Could you check a few things on this model? Use its own coordinates, in mm. Round coordinates to 2 decimals unless told otherwise and drop trailing zeros. Loops run counter-clockwise (first coordinate to the right, second up) from the corner with the lowest first, then second, coordinate; pieces in that order, holes last. Notation, with made-up numbers: (89, 9) -> (94, 9) arc R29 ccw to (94, 30) -> close; hole circle Ø10 at (28, 34). An arc over 180 degrees is marked (long way). Write each question's results on one line, items separated by ' | '.
from build123d import *

# Parameters (mm, degrees)
SKETCH_W      = 12
SKETCH_H      = 45
PAD_DEPTH     = 5
SKETCH001_R   = 2.2
SKETCH001_R_2 = 2
POCKET_DEPTH  = 5.001
CHAMFER_SIZE2 = 12
CHAMFER_SIZE  = 3
FILLET_R      = 3
FILLET001_R   = 5.5


with BuildPart() as part:
    # Sketch → Pad (new body)
    with BuildSketch(Plane.XY):
        Rectangle(SKETCH_W, SKETCH_H)
    extrude(amount=PAD_DEPTH)

    # Sketch001 (on Face6 of Pad) → Pocket (cut, through all)
    with BuildSketch(Plane.XY.offset(5)):
        with Locations((0, 17)):
            Circle(SKETCH001_R)
        with Locations((-0.5, -16.5)):
            Circle(SKETCH001_R_2)
        with Locations((-0.5, -4.5)):
            Circle(SKETCH001_R_2)
    extrude(amount=-POCKET_DEPTH, mode=Mode.SUBTRACT)

    # Chamfer
    chamfer_edges = [part.edges().sort_by_distance(p)[0] for p in [
        (6, -22.5, 2.5),
    ]]
    chamfer_side = part.faces().sort_by_distance((0, -22.5, 2.5))[0]
    chamfer(chamfer_edges, length=CHAMFER_SIZE, length2=CHAMFER_SIZE2, reference=chamfer_side)

    # Fillet
    fillet_edges = [part.edges().sort_by_distance(p)[0] for p in [
        (3, -22.5, 2.5),
    ]]
    fillet(fillet_edges, radius=FILLET_R)

    # Fillet001
    fillet001_edges = [part.edges().sort_by_distance(p)[0] for p in [
        (6, 22.5, 2.5),
        (-6, 22.5, 2.5),
    ]]
    fillet(fillet001_edges, radius=FILLET001_R)


solid = part.part
1) I want a section at B-B, the plane z = 4.45. Write out the boundary of the cut face in (x, y), plus the area to 3 significant figures.
Model answer:
outline: (-6, -22.5) -> (0.66, -22.5) arc R3 ccw to (3.57, -20.23) -> (6, -10.5) -> (6, 17) arc R5.5 ccw to (0.5, 22.5) -> (-0.5, 22.5) arc R5.5 ccw to (-6, 17) -> close; hole circle Ø4 at (-0.5, -16.5); hole circle Ø4 at (-0.5, -4.5); hole circle Ø4.4 at (0, 17) | area: 468 mm2
2) I want a section at D-D, the plane x = 4.25. Write out the boundary of the cut face in (y, z).
Model answer:
outline: (-17.5, 0) -> (21.02, 0) -> (21.02, 5) -> (-17.5, 5) -> close
3) I need wall thicknesses on line 1 (Y direction, x = 0, z = 1.45); line 2 (Y direction, x = -0.5, z = 3.85); line 3 (X direction, y = -16, z = 4.4) (1 decimal). Which ranges of each line are inside material? Lowest first, please.
Model answer:
line 1: y = -22.5 to -18.44, -14.56 to -6.44, -2.56 to 14.8, 19.2 to 22.5 | line 2: y = -22.5 to -18.5, -14.5 to -6.5, -2.5 to 14.86, 19.14 to 22.5 | line 3: x = -6 to -2.4, 1.4 to 4.6
4) I want a section at A-A, the plane y = -16.5. Write out the boundary of the cut face in (x, z), plus the area to 3 significant figures.
Model answer:
outline: (-6, 0) -> (-2.5, 0) -> (-2.5, 5) -> (-6, 5) -> close; (1.5, 0) -> (4.5, 0) -> (4.5, 5) -> (1.5, 5) -> close | area: 32.5 mm2
5) I'm going to push a flat-ended pin straight in: pin 1 (3 mm diameter, centred on y = -15.5, z = 1, fed in from +X) (3 decimals). Where does the tip first touch, or does it pass through?
Model answer:
pin 1: stops at x = 5.125
6) I want a section at C-C, the plane y = -4.5. Write out the boundary of the cut face in (x, z).
Model answer:
outline: (-6, 0) -> (-2.5, 0) -> (-2.5, 5) -> (-6, 5) -> close; (1.5, 0) -> (6, 0) -> (6, 5) -> (1.5, 5) -> close
7) If we mould it in two halves opening along Y, with no side actions, what happens to faces 1 (the flat face through (6, 3, 2)), 2 (the flat face through (-3, -22.5, 2)), 3 (the cylindrical face through (-0.76, -14.517, 2.535))? For each: released by +Y, released by -Y, zero draft, split by the parting line, or undercut.
Model answer:
face 1: zero draft | face 2: released by -Y | face 3: undercut
